Geometry: final body of the model. Coordinates: model frame, mm. A direction names the side the tool comes from. Round coordinates to 2 decimals unless told otherwise and drop trailing zeros. Write each loop counter-clockwise with the first axis right and the second up, starting at its lowest first coordinate (ties: lowest second). Pieces come first, ordered by that corner, then holes. Notation, with made-up numbers: M 20,4 L 62,4 A27 cw 62,28 Z; hole C 11.5,37 d1. An arc over 180 degrees is marked long. Answer as CSV lines item,"result". Start each with the question number.
Q1. Section query D-D on z = 3.2. Give the number of separate pieces and of enclosed holes in the cut face, and give its area (3 significant figures).
Q2. Mould query, pull axis Y, two halves, no side actions, for faces 3 (the flat face through (0, 40, 2)), 4 (the cylindrical face through (-36.6, 0, 2)), 5 (the flat face through (-18, 1, 0)), 6 (the flat face through (-27, 1.6, 2)). Classes: pulls with the +Y half, pulls with the -Y half, needs draft (parallel to the pull), parting line crosses it, or undercut.
Q3. Ray query, probe 1 along X at (y, z) = (21, 3.2); probe 2 along X at (y, z) = (24, 3.3); probe 3 along Y at (x, z) = (2, 2.15). Return the intervals inside material, ascending.
Q4. Reachability of faces 1 (the cylindrical face through (0, -36.6, 2)), 2 (the cylindrical face through (38, 39, 2)) from +Z, -Z, +X, -X, +Y, -Y: full face, straight path, thin tool, end or side. Return the list, or none.
Q5. Section query B-B on y = 0. Output: boundary loops of the cut face in (x, z).
Q6. Section query A-A on y = -32.5. Output: boundary loops of the cut face in (x, z).
Q7. First-contact query: pin 1 (2.5 mm diameter, centred on x = 20.86, y = 20.86, fed in from +Z). Flat tip, straight axial feed; report the tip coordinate or a pass-through.
```python
from build123d import *

# Parameters (mm, degrees)
SKETCH2_W           = 80
SKETCH2_H           = 80
SKETCH2_R           = 1.575
BOSS_EXTRUDE1_DEPTH = 4
FILLET1_R           = 5


with BuildPart() as part:
    # Sketch2 → Boss-Extrude1 (new body)
    with BuildSketch(Plane.XY):
        Rectangle(SKETCH2_W, SKETCH2_H)
        with Locations((-20.859650045, -20.859650045)):
            Circle(SKETCH2_R, mode=Mode.SUBTRACT)
        with Locations((-20.859650045, 20.859650045)):
            Circle(SKETCH2_R, mode=Mode.SUBTRACT)
        with Locations((20.859650045, 20.859650045)):
            Circle(SKETCH2_R, mode=Mode.SUBTRACT)
        with Locations((20.859650045, -20.859650045)):
            Circle(SKETCH2_R, mode=Mode.SUBTRACT)
        with BuildLine():
            Line((1.6, 20), (1.6, 35))
            ThreePointArc((1.6, 35), (1.13137085, 36.13137085), (0, 36.6))
            ThreePointArc((0, 36.6), (-1.13137085, 36.13137085), (-1.6, 35))
            Line((-1.6, 35), (-1.6, 20))
            ThreePointArc((-1.6, 20), (0, 18.4), (1.6, 20))
        make_face(mode=Mode.SUBTRACT)
        with BuildLine():
            Line((1.6, -35), (1.6, -20))
            ThreePointArc((1.6, -20), (1.13137085, -18.86862915), (0, -18.4))
            ThreePointArc((0, -18.4), (-1.13137085, -18.86862915), (-1.6, -20))
            Line((-1.6, -20), (-1.6, -35))
            ThreePointArc((-1.6, -35), (0, -36.6), (1.6, -35))
        make_face(mode=Mode.SUBTRACT)
        with BuildLine():
            Line((20, -1.6), (35, -1.6))
            ThreePointArc((35, -1.6), (36.6, 0), (35, 1.6))
            Line((35, 1.6), (20, 1.6))
            ThreePointArc((20, 1.6), (18.4, 0), (20, -1.6))
        make_face(mode=Mode.SUBTRACT)
        with BuildLine():
            Line((-35, -1.6), (-20, -1.6))
            ThreePointArc((-20, -1.6), (-18.4, 0), (-20, 1.6))
            Line((-20, 1.6), (-35, 1.6))
            ThreePointArc((-35, 1.6), (-36.6, 0), (-35, -1.6))
        make_face(mode=Mode.SUBTRACT)
        with BuildLine():
            ThreePointArc((0, -14), (14, 0), (0, 14))
            ThreePointArc((0, 14), (-14, 0), (0, -14))
        make_face(mode=Mode.SUBTRACT)
    extrude(amount=BOSS_EXTRUDE1_DEPTH)

    # Fillet1
    fillet1_edges = [part.edges().sort_by_distance(p)[0] for p in [
        (40, -40, 2),
        (-40, -40, 2),
        (-40, 40, 2),
        (40, 40, 2),
    ]]
    fillet(fillet1_edges, radius=FILLET1_R)


solid = part.part
```
Entries:
1,separate pieces,"1"
1,enclosed holes,"9"
1,area,"5,510 mm^2"
2,face 3,"pulls with the +Y half"
2,face 4,"undercut"
2,face 5,"needs draft"
2,face 6,"undercut"
3,probe 1,"x = -40 to -22.43, -19.29 to -1.6, 1.6 to 19.29, 22.43 to 40"
3,probe 2,"x = -40 to -1.6, 1.6 to 40"
3,probe 3,"y = -40 to -13.86, 13.86 to 40"
4,face 1,"+Z, -Z"
4,face 2,"+Z, -Z, +X, +Y"
5,outline,"M -40,0 L -36.6,0 L -36.6,4 L -40,4 Z; M -18.4,0 L -14,0 L -14,4 L -18.4,4 Z; M 14,0 L 18.4,0 L 18.4,4 L 14,4 Z; M 36.6,0 L 40,0 L 40,4 L 36.6,4 Z"
6,outline,"M -40,0 L -1.6,0 L -1.6,4 L -40,4 Z; M 1.6,0 L 40,0 L 40,4 L 1.6,4 Z"
7,pin 1,"passes through"
